For this review, take the finished solid that the model builds, in its own axes (mm). A direction names the side the tool comes from. Coordinates: 2 decimals unless noted, no trailing zeros. Loops run counter-clockwise (first coordinate to the right, second up) from the corner with the lowest first, then second, coordinate; pieces in that order, holes last. Notation, with made-up numbers: (33.5, -29) - (91.5, -29) arc R12 cw to (91.5, -23) - close; hole circle Ø11 at (-20, 46). An arc over 180 degrees is marked (long way). Answer as a JSON object with one key per item and string values. Group by question number.
Item 1: Clearance check with flat-ended pins moving along their axes: pin 1 (3 mm diameter, centred on y = 2.9, z = 13.6, fed in from -X); pin 2 (1.5 mm diameter, centred on y = 3.5, z = -8.5, fed in from +X); pin 3 (2.5 mm diameter, centred on y = 2.9, z = 13.6, fed in from -X); pin 4 (2 mm diameter, centred on y = 5, z = 8.5, fed in from -X). State where each tip first meets the part, or that it passes through.
Item 2: To check wall thickness, follow line 1 (X direction, y = 1.3, z = 12.5); line 2 (X direction, y = 1.45, z = 4); line 3 (Y direction, x = 59.25, z = 13.6). State the ranges of each line that lie inside material, in increasing order.
Item 3: We need section A-A (z = 5.5). Give the boundary of the cut face in (x, y).
Item 4: Mouldability with a two-part tool opening along Z and no side actions: class faces 4 (the flat face through (56, 3, 14)), 5 (the flat face through (-74, 3, 8.1)), 6 (the flat face through (-71, 3, -7)) as released by +Z, released by -Z, zero draft, split by the parting line, or undercut.
Item 5: We need section B-B (x = 43.5). Give the boundary of the cut face in (y, z), then the cut area to 3 significant figures.
Item 6: Tool access review of faces 1 (the flat face through (-64.9, 4.4, 13.6)), 2 (the cylindrical face through (-69.077, 4.038, 14.326)), 3 (the flat face through (74, 3, 8.1)): name each direction out of +Z, -Z, +X, -X, +Y, -Y from which nothing blocks a thin tool from reaching the whole face with its end or side.
Autodesk Inventor part; units mm, degrees
ref_plane "우측면도" through (0, 0, 0) normal (1, 0, 0) x (0, 1, 0)
ref_plane "평면도" through (0, 0, 0) normal (0, 1, 0) x (-1, 0, 0)
ref_plane "정면도" through (0, 0, 0) normal (0, 0, 1) x (1, 0, 0)
sketch "스케치1" plane through (0, 0, 0) normal (0, 1, 0) x (-1, 0, 0)
  line L0 (-71, 24.6) -> (71, 24.6)
  line L1 (71, 24.6) -> (71, -10)
  line L2 (-71, -10) -> (-71, 24.6)
  line L3 (-71, 24.6) -> (71, -24.6) construction
  line L4 (71, 24.6) -> (-71, -24.6) construction
  line L5 (-71, 8.1) -> (-77, 8.1)
  line L6 (-77, 8.1) -> (-77, -3.9)
  line L7 (-77, -3.9) -> (-71, -3.9)
  line L8 (-71, -3.9) -> (-71, 8.1)
  line L9 (71, 8.1) -> (77, 8.1)
  line L10 (77, 8.1) -> (77, -3.9)
  line L11 (77, -3.9) -> (71, -3.9)
  line L12 (71, -3.9) -> (71, 8.1)
  line L13 (27.5, 10) -> (-27.5, 10)
  line L14 (-27.5, 10) -> (-27.5, -10)
  line L15 (-27.5, -10) -> (27.5, -10)
  line L16 (27.5, -10) -> (27.5, 10)
  line L17 (27.5, 10) -> (-27.5, -10) construction
  line L18 (-27.5, 10) -> (27.5, -10) construction
  line L19 (27.5, -10) -> (71, -10)
  line L20 (-27.5, -10) -> (-71, -10)
  line L21 (71, -24.6) -> (67.65, -24.6)
  line L22 (-67.65, -24.6) -> (-71, -24.6)
  point P0 (0, 0)
  dimension "d0" = 142
  dimension "d1" = 49.2
  dimension "d2" = 6
  dimension "d3" = 12
  dimension "d4" = 6
  dimension "d5" = 55
  dimension "d6" = 20
extrude "돌출2" add sketch "스케치1" along normal blind 6 contours L0 L1 L19 L16 L13 L14 L20 L2 | L2 L7 L6 L5 | L9 L10 L11 L1
sketch "스케치2" plane through (0, 6, 0) normal (0, 1, 0) x (1, 0, 0)
  line L0 (-50, 10) -> (50, 10)
  line L1 (50, 10) -> (50, -10)
  line L2 (50, -10) -> (-50, -10)
  line L3 (-50, -10) -> (-50, 10)
  line L4 (-50, 10) -> (50, -10) construction
  line L5 (50, 10) -> (-50, -10) construction
  point P0 (0, 0)
  dimension "d11" = 100
  dimension "d12" = 20
extrude "돌출3" cut sketch "스케치2" against normal blind 6
sketch "스케치3" plane through (71, 0, 24.6) normal (1, 0, 0) x (0, 0, -1)
  circle A0 centre (11, 2.9) radius 1.35
  circle A1 centre (11, 2.9) radius 1.35
  point P0 (24.6, 0)
extrude "돌출4" cut sketch "스케치3" against normal blind 15
sketch "스케치4" plane through (-71, 0, 8.1) normal (-1, 0, 0) x (0, 0, 1)
  circle A0 centre (5.5, 2.9) radius 1.35
  circle A1 centre (5.5, 2.9) radius 1.35
  point P0 (-8.1, 0)
extrude "돌출5" cut sketch "스케치4" against normal blind 15
sketch "스케치5" plane through (0, 6, 0) normal (0, 1, 0) x (1, 0, 0)
  line L0 (71, -12.25) -> (56, -12.25)
  line L1 (71, -14.95) -> (56, -14.95)
  line L2 (-71, -12.25) -> (-56, -12.25)
  line L3 (-71, -14.95) -> (-56, -14.95)
  line L4 (-66, -12.25) -> (-66, -14.95)
  line L5 (66, -12.25) -> (66, -14.95)
  line L6 (-67.1, -16.2) -> (-64.9, -16.2)
  line L7 (-64.9, -16.2) -> (-64.9, -11)
  line L8 (-64.9, -11) -> (-67.1, -11)
  line L9 (-67.1, -11) -> (-67.1, -16.2)
  line L10 (-67.1, -16.2) -> (-64.9, -11) construction
  line L11 (-64.9, -16.2) -> (-67.1, -11) construction
  line L12 (67.1, -16.2) -> (64.9, -16.2)
  line L13 (64.9, -16.2) -> (64.9, -11)
  line L14 (64.9, -11) -> (67.1, -11)
  line L15 (67.1, -11) -> (67.1, -16.2)
  line L16 (67.1, -16.2) -> (64.9, -11) construction
  line L17 (64.9, -16.2) -> (67.1, -11) construction
  point P0 (0, 0)
  point P1 (-66, -13.6)
  point P2 (66, -13.6)
  dimension "d19" = 2.2
  dimension "d20" = 5.2
  dimension "d21" = 2.2
  dimension "d22" = 5.2
extrude "돌출6" cut sketch "스케치5" against normal blind 15
sketch "스케치6" plane through (0, 6, 0) normal (0, 1, 0) x (1, 0, 0)
  line L0 (67.1, -11) -> (67.1, -16.2)
  line L1 (67.1, -16.2) -> (64.9, -16.2)
  line L2 (64.9, -16.2) -> (64.9, -11)
  line L3 (64.9, -11) -> (67.1, -11)
  line L4 (-67.1, -16.2) -> (-67.1, -11)
  line L5 (-67.1, -11) -> (-64.9, -11)
  line L6 (-64.9, -11) -> (-64.9, -16.2)
  line L7 (-64.9, -16.2) -> (-67.1, -16.2)
  line L8 (-50, -10) -> (-50, 10)
  line L9 (-50, 10) -> (-71, 10)
  line L10 (-71, 10) -> (-71, 3.9)
  line L11 (-71, 3.9) -> (-77, 3.9)
  line L12 (-77, 3.9) -> (-77, -8.1)
  line L13 (-77, -8.1) -> (-71, -8.1)
  line L14 (-71, -8.1) -> (-71, -24.6)
  line L15 (-71, -24.6) -> (71, -24.6)
  line L16 (71, -24.6) -> (71, -8.1)
  line L17 (71, -8.1) -> (77, -8.1)
  line L18 (77, -8.1) -> (77, 3.9)
  line L19 (77, 3.9) -> (71, 3.9)
  line L20 (71, 3.9) -> (71, 10)
  line L21 (71, 10) -> (50, 10)
  line L22 (50, 10) -> (50, -10)
  line L23 (50, -10) -> (-50, -10)
  line L24 (-55, -10) -> (55, -10)
  line L25 (55, -10) -> (55, 10)
  line L26 (55, 10) -> (-55, 10)
  line L27 (-55, 10) -> (-55, -10)
  line L28 (-55, -10) -> (55, 10) construction
  line L29 (55, -10) -> (-55, 10) construction
  point P0 (0, 0)
  dimension "d25" = 110
extrude "돌출8" cut sketch "스케치6" against normal blind 10 contours L24 L27 L9 L8 | L22 L21 L25 L24
sketch "스케치7" plane through (0, 6, 0) normal (0, 1, 0) x (1, 0, 0)
  line L0 (-67.1, -16.2) -> (-67.1, -11)
  line L1 (-67.1, -11) -> (-64.9, -11)
  line L2 (-64.9, -11) -> (-64.9, -16.2)
  line L3 (-64.9, -16.2) -> (-67.1, -16.2)
  line L4 (67.1, -11) -> (67.1, -16.2)
  line L5 (67.1, -16.2) -> (64.9, -16.2)
  line L6 (64.9, -16.2) -> (64.9, -11)
  line L7 (64.9, -11) -> (67.1, -11)
  line L8 (55, 10) -> (55, -10)
  line L9 (55, -10) -> (-55, -10)
  line L10 (-55, -10) -> (-55, 10)
  line L11 (-55, 10) -> (-71, 10)
  line L12 (-71, 10) -> (-71, 3.9)
  line L13 (-71, 3.9) -> (-77, 3.9)
  line L14 (-77, 3.9) -> (-77, -8.1)
  line L15 (-77, -8.1) -> (-71, -8.1)
  line L16 (-71, -8.1) -> (-71, -24.6)
  line L17 (-71, -24.6) -> (71, -24.6)
  line L18 (71, -24.6) -> (71, -8.1)
  line L19 (71, -8.1) -> (77, -8.1)
  line L20 (77, -8.1) -> (77, 3.9)
  line L21 (77, 3.9) -> (71, 3.9)
  line L22 (71, 3.9) -> (71, 10)
  line L23 (71, 10) -> (55, 10)
  circle A0 centre (-71, 3.9) radius 1
  circle A1 centre (-71, -8.1) radius 1
  circle A2 centre (71, -8.1) radius 1
  circle A3 centre (71, 3.9) radius 1
  point P0 (0, 0)
  point P1 (72, -8.1)
  point P2 (71, -9.1)
  point P3 (71, 4.9)
  point P4 (72, 3.9)
  point P5 (-71, 4.9)
  point P6 (-72, 3.9)
  point P7 (-71, -9.1)
  point P8 (-72, -8.1)
  dimension "d30" = 2
  dimension "d31" = 2
  dimension "d32" = 2
  dimension "d33" = 2
extrude "돌출9" cut sketch "스케치7" against normal blind 10 contours L22 L21 A3 | A0 L13 L12 | L19 L18 A2 | A1 L16 L15 picked at (71.1358, 3.2525) picked at (-71.657, 3.8202) picked at (71.1358, -7.4525) picked at (-71, -7.4382)
properties part number "battery backplate" material "PMMA 플라스틱"
Check sheet entries:
{
 "1": {"pin 1": "stops at x = -71", "pin 2": "stops at x = 71", "pin 3": "stops at x = -56", "pin 4": "stops at x = -77"},
 "2": {"line 1": "x = -71 to -67.1, -64.9 to 64.9, 67.1 to 71", "line 2": "x = -77 to -55, 55 to 77", "line 3": "y = 0 to 1.55, 4.25 to 6"},
 "3": {"outline": "(-77, 0) - (-55, 0) - (-55, 6) - (-77, 6) - close; (55, 0) - (77, 0) - (77, 6) - (55, 6) - close"},
 "4": {"face 4": "undercut", "face 5": "released by +Z", "face 6": "zero draft"},
 "5": {"outline": "(0, 10) - (6, 10) - (6, 24.6) - (0, 24.6) - close", "area": "87.6 mm2"},
 "6": {"face 1": "+Y, -Y", "face 2": "-X", "face 3": "+Z, +X, +Y, -Y"}
}
